from build123d import *

# Parameters (mm, degrees)
ESQUISSE1_R                         = 7.5
BOSS_EXTRU_1_DEPTH                  = 5
CONG_1_R                            = 1
ESQUISSE12_W                        = 4.75
ESQUISSE12_H                        = 42
CONG_2_R                            = 1
ENL_V_START                         = -4.7500001
ENL_V_DE_MAT_R_VOL_MINCE2_OUTLINE_R = 1.5
ENL_V_DE_MAT_R_VOL_MINCE2_DEPTH     = 9.5000002


# Read off the part's stored shape, not the designer's step: Enlèv. de mat.-Révol.-Mince2
with BuildPart() as part:
    # Esquisse1 → Boss.-Extru.1 (new body)
    with BuildSketch(Plane.XY):
        Circle(ESQUISSE1_R)
    extrude(amount=BOSS_EXTRU_1_DEPTH)

    # Congé1
    cong_1_edges = [part.edges().sort_by_distance(p)[0] for p in [
        (-7.5, 0, 5),
    ]]
    fillet(cong_1_edges, radius=CONG_1_R)

    # Esquisse12 → Révolution1 (revolve)
    with BuildSketch(Plane(origin=(0, 0, 0), x_dir=(1, 0, 0), z_dir=(0, 1, 0))):
        with Locations((2.375, 21)):
            Rectangle(ESQUISSE12_W, ESQUISSE12_H)
    revolve(axis=Axis((0, 0, 0), (0, 0, -1)))

    # Congé2
    cong_2_edges = [part.edges().sort_by_distance(p)[0] for p in [
        (-4.75, 0, -42),
    ]]
    fillet(cong_2_edges, radius=CONG_2_R)

    # Enlèv. de mat.-Révol.-Mince2 outline → Enlèv. de mat.-Révol.-Mince2 (cut)
    with BuildSketch(Plane.YZ.offset(ENL_V_START)):
        with Locations((0, -37)):
            Circle(ENL_V_DE_MAT_R_VOL_MINCE2_OUTLINE_R)
    extrude(amount=ENL_V_DE_MAT_R_VOL_MINCE2_DEPTH, mode=Mode.SUBTRACT)


solid = part.part
For this review, take the finished solid that the model builds, in its own axes (mm). A direction names the side the tool comes from. Round coordinates to 2 decimals unless told otherwise and drop trailing zeros. Write each loop counter-clockwise with the first axis right and the second up, starting at its lowest first coordinate (ties: lowest second). Pieces come first, ordered by that corner, then holes. Notation, with made-up numbers: (-12, 68.25) -> (13, 68.25) arc R25 cw to (13, 80.25) -> close; hole circle Ø6 at (77, 4.25). An arc over 180 degrees is marked (long way). Put each result on its own line as item: value.
Q1. The part is to be moulded in two halves that separate along Y. For faces 1 (the cylindrical face through (-7.493, 0.33, 1.972)), 2 (the flat face through (0, 0, 5)), 3 (the cylindrical face through (-0.067, -0.325, -38.464)), say which applies: released by +Y, released by -Y, zero draft, split by the parting line, or undercut.
Determined:
face 1: split by the parting line
face 2: zero draft
face 3: undercut
Q2. To check wall thickness, follow L1, parallel to Z at x = -2.5, y = 0; L2, parallel to Y at x = 0.5, z = -37; L3, parallel to Y at x = 3.75, z = -37.5. State the ranges of each line that lie inside material, in increasing order. Write a range as [from, to].
Determined:
L1: z = [-42, -38.5], [-35.5, 5]
L2: y = [-4.72, -1.5], [1.5, 4.72]
L3: y = [-2.92, -1.41], [1.41, 2.92]
Q3. Consider section B-B on z = -29. State the section outline as (x, y) points.
Determined:
outline: circle Ø9.5 at (0, 0)
Q4. Machinability: for faces 4 (the cylindrical face through (2.192, 4.214, -20.787)), 5 (the flat face through (0, 0, -42)), which of the approach directions +Z, -Z, +X, -X, +Y, -Y give a long, thin tool a straight path to every point of the face, cutting with its end or side? Answer none if there is none.
Determined:
face 4: -Z
face 5: -Z, +X, -X, +Y, -Y
Q5. Clearance check with flat-ended pins moving along their axes: pin 1 Ø3 at (x, z) = (-1.5, -31) entering from -Y; pin 2 Ø8 at (x, y) = (-5.5, 3) entering from -Z; pin 3 Ø2 at (y, z) = (-3.5, -26.5) entering from -X; pin 4 Ø1 at (y, z) = (2, -24.5) entering from -X. State where each tip first meets the part, or that it passes through.
Determined:
pin 1: stops at y = -4.75
pin 2: stops at z = -42
pin 3: stops at x = -4.04
pin 4: stops at x = -4.51
Q6. Consider section C-C on z = -37. State the section outline as (x, y) points.
Determined:
outline: (-4.51, -1.5) arc R4.75 ccw to (4.51, -1.5) -> close; (-4.51, 1.5) -> (4.51, 1.5) arc R4.75 ccw to start
Q7. Consider section A-A on y = 0. State the section outline as (x, z) points, and give its area (3 significant figures).
Determined:
outline: (-7.5, 0) -> (-4.75, 0) -> (-4.75, -35.5) -> (4.75, -35.5) -> (4.75, 0) -> (7.5, 0) -> (7.5, 4) arc R1 ccw to (6.5, 5) -> (-6.5, 5) arc R1 ccw to (-7.5, 4) -> close; (-4.75, -41) arc R1 ccw to (-3.75, -42) -> (3.75, -42) arc R1 ccw to (4.75, -41) -> (4.75, -38.5) -> (-4.75, -38.5) -> close
area: 445 mm^2
